Design review of the part built by this model. Coordinates are the model's own, in mm. A direction names the side the tool comes from. Round coordinates to 2 decimals unless told otherwise and drop trailing zeros. Order: outer loops, then holes, each group sorted by start corner. A loop starts at its lowest first (then second) coordinate and runs counter-clockwise, first axis right, second up. Notation, with made-up numbers: (20, 5) - (45, 5) arc R30 ccw to (45, 35) - close; hole circle Ø11 at (46.5, 19.5). An arc over 180 degrees is marked (long way). Use CSV: the item, a comma, the result in double quotes.
from build123d import *

# Parameters (mm, degrees)
SKETCH1_R           = 70
SKETCH1_R_2         = 44.35
BOSS_EXTRUDE1_DEPTH = 8.6
SKETCH2_R           = 58.5
SKETCH2_R_2         = 57.5
CUT_EXTRUDE1_DEPTH  = 2
SKETCH3_R           = 2.7
CUT_EXTRUDE2_DEPTH  = 9.6
SKETCH4_R           = 2.7
CUT_EXTRUDE3_DEPTH  = 9.6


with BuildPart() as part:
    # Sketch1 → Boss-Extrude1 (new body)
    with BuildSketch(Plane(origin=(0, 0, 0), x_dir=(1, 0, 0), z_dir=(0, 1, 0))):
        Circle(SKETCH1_R)
        Circle(SKETCH1_R_2, mode=Mode.SUBTRACT)
    extrude(amount=BOSS_EXTRUDE1_DEPTH)

    # Sketch2 → Cut-Extrude1 (cut)
    with BuildSketch(Plane(origin=(0, 8.6, 0), x_dir=(1, 0, 0), z_dir=(0, 1, 0))):
        Circle(SKETCH2_R)
        Circle(SKETCH2_R_2, mode=Mode.SUBTRACT)
    cut_extrude1 = extrude(amount=-CUT_EXTRUDE1_DEPTH, mode=Mode.SUBTRACT)

    # Mirror1: Cut-Extrude1 across plane
    add(cut_extrude1.mirror(Plane.ZX.offset(4.3)), mode=Mode.SUBTRACT)

    # Sketch3 → Cut-Extrude2 (cut, through all)
    with BuildSketch(Plane(origin=(0, 8.6, 0), x_dir=(1, 0, 0), z_dir=(0, 1, 0))):
        with Locations((0, 64.25)):
            Circle(SKETCH3_R)
        with Locations((64.25, 0)):
            Circle(SKETCH3_R)
        with Locations((0, -64.25)):
            Circle(SKETCH3_R)
        with Locations((-64.25, 0)):
            Circle(SKETCH3_R)
    extrude(amount=-CUT_EXTRUDE2_DEPTH, mode=Mode.SUBTRACT)

    # Sketch4 → Cut-Extrude3 (cut, through all)
    with BuildSketch(Plane(origin=(0, 8.6, 0), x_dir=(1, 0, 0), z_dir=(0, 1, 0))):
        with Locations((-36.009412832, 36.009412832)):
            Circle(SKETCH4_R)
        with Locations((36.009412832, 36.009412832)):
            Circle(SKETCH4_R)
        with Locations((36.009412832, -36.009412832)):
            Circle(SKETCH4_R)
        with Locations((-36.009412832, -36.009412832)):
            Circle(SKETCH4_R)
    extrude(amount=-CUT_EXTRUDE3_DEPTH, mode=Mode.SUBTRACT)


solid = part.part
1) We need section A-A (x = 0). Give the number of separate pieces and of enclosed holes in the cut face, then the cut area to 3 significant figures.
Data:
separate pieces,"4"
enclosed holes,"0"
area,"340 mm2"
2) For faces 1 (the face through (43, 6.6, 39)), 2 (the face through (-12.68, 0.99, 57.11)), 3 (the face through (-0.585, 4.36, -61.614)), list the 3-axis set-ups (+Z, -Z, +X, -X, +Y, -Y) from which the entire face can be reached by the end or side of a thin tool; tool diameter is ignored.
Data:
face 1,"+Y"
face 2,"-Y"
face 3,"+Y, -Y"
3) To check wall thickness, follow L1, parallel to X at y = 7.25, z = 0; L2, parallel to Z at x = 10.5, y = 8.25; L3, parallel to X at y = 2.5, z = -2. State the ranges of each line that lie inside material, in increasing order. Write a range as from..to.
Data:
L1,"x = -70..-66.95, -61.55..-58.5, -57.5..-44.35, 44.35..57.5, 58.5..61.55, 66.95..70"
L2,"z = -69.21..-57.55, -56.53..-43.09, 43.09..56.53, 57.55..69.21"
L3,"x = -69.97..-66.06, -62.44..-44.3, 44.3..62.44, 66.06..69.97"
4) We need section C-C (x = -30). Give the boundary of the cut face in (y, z), then the cut area to 3 significant figures.
Data:
outline,"(0, -63.25) - (8.6, -63.25) - (8.6, -50.22) - (6.6, -50.22) - (6.6, -49.05) - (8.6, -49.05) - (8.6, -32.66) - (0, -32.66) - (0, -49.05) - (2, -49.05) - (2, -50.22) - (0, -50.22) - close; (0, 32.66) - (8.6, 32.66) - (8.6, 49.05) - (6.6, 49.05) - (6.6, 50.22) - (8.6, 50.22) - (8.6, 63.25) - (0, 63.25) - (0, 50.22) - (2, 50.22) - (2, 49.05) - (0, 49.05) - close"
area,"517 mm2"
5) We need section D-D (z = 64.25). Give the boundary of the cut face in (x, y), then the cut area to 3 significant figures.
Data:
outline,"(-27.78, 0) - (-2.7, 0) - (-2.7, 8.6) - (-27.78, 8.6) - close; (2.7, 0) - (27.78, 0) - (27.78, 8.6) - (2.7, 8.6) - close"
area,"431 mm2"
6) The part is to be moulded in two halves that separate along X. For faces 4 (the face through (43, 2, 39)), 5 (the face through (30, 0, 34)), 6 (the face through (-55.55, 4.24, 42.594)), say which applies: +X half, -X half, draft (parallel to the pull), parting line (faces both ways), or undercut.
Data:
face 4,"undercut"
face 5,"draft"
face 6,"parting line"
7) Insertion check: pin 1 Ø4.5 at (x, z) = (-64.25, 0) entering from +Y; pin 2 Ø5 at (y, z) = (5.5, 22.5) entering from +X; pin 3 Ø3 at (x, y) = (-19, 2.5) entering from +Z; pin 4 Ø2 at (y, z) = (4.5, -12) entering from -X. Each pin has a flat end and moves straight along its axis. Give the tip position at first contact, or say it passes through.
Data:
pin 1,"passes through"
pin 2,"stops at x = 67.08"
pin 3,"stops at z = 67.78"
pin 4,"stops at x = -69.13"
